Autodesk Inventor part; units mm, degrees
ref_plane "YZ Plane" through (0, 0, 0) normal (1, 0, 0) x (0, 1, 0)
ref_plane "XZ Plane" through (0, 0, 0) normal (0, 1, 0) x (-1, 0, 0)
ref_plane "XY Plane" through (0, 0, 0) normal (0, 0, 1) x (1, 0, 0)
sketch "スケッチ1" plane through (0, 0, 0) normal (0, 0, 1) x (1, 0, 0)
  line L0 (0, 25) -> (-3.75, 25)
  line L1 (-3.75, 25) -> (-3.75, 0)
  line L2 (-3.75, 0) -> (0, 0)
  line L3 (0, 0) -> (0, 25)
  line L4 (0, -5) -> (0, 30)
  line L5 (-4.5, 0) -> (0.75, 0)
  dimension "d2" = 3.75
  dimension "d3" = 25
revolve "回転1" add sketch "スケッチ1" angle 360 about axis through (0, -10, 0) along (0, 1, 0)
sketch "スケッチ3" plane through (0, 25, 0) normal (0, 1, 0) x (1, 0, 0)
  circle A0 centre (0, 0) radius 2.5
  dimension "d5" = 5
extrude "押し出し1" cut sketch "スケッチ3" against normal blind 5
sketch "スケッチ4" plane through (0, 0, 0) normal (0, -1, 0) x (1, 0, 0)
  circle A0 centre (0, 0) radius 3.75
  line L0 (3.75, 3.25) -> (5.75, 3.25)
  line L1 (3.75, -3.25) -> (5.75, -3.25)
  line L2 (5.75, -3.25) -> (5.75, 3.25)
  line L3 (2.7951, 2.5) -> (3.75, 2.5)
  line L4 (-5.65, 0) -> (7.65, 0)
  line L5 (3.75, 3.25) -> (3.75, 2.5)
  line L6 (3.75, 0) -> (3.75, -3.25)
  line L7 (2.7951, -2.5) -> (3.75, -2.5)
  dimension "d9" = 6.5
  dimension "d10" = 2
  dimension "d11" = 2.5
  dimension "d12" = 5
extrude "押し出し2" add sketch "スケッチ4" against normal blind 20 contours L6 L7 A0 | A0 L3 L5 L0 L2 L4 | L4 L2 L1 L6
fillet "フィレット1" radius 0.5 4 edges at (5.75, 10, 3.25) (5.75, 10, -3.25) (3.75, 10, 3.25) (3.75, 10, -3.25)
properties part number "flat_cover_5mm"
Geometry: final body of the model. Coordinates: model frame, mm. A direction names the side the tool comes from. Give positions to 0.01 mm unless a question says otherwise; leave off trailing zeros. Loops run counter-clockwise (first coordinate to the right, second up) from the corner with the lowest first, then second, coordinate; pieces in that order, holes last. Notation, with made-up numbers: (7, 7.5) -> (19, 7.5) arc R18 ccw to (19, 32.5) -> close; hole circle Ø5 at (-15.75, -18). An arc over 180 degrees is marked (long way). Put each result on its own line as item: value.
1. Pin query (flat end, axial travel): P1, Ø0.8, axis at x = 4.5, y = 5.5, coming from the +Z side; P2, Ø2.5, axis at x = 0, z = 1, coming from the +Y side; P3, Ø1.1, axis at x = 4.5, y = 7.5, coming from the -Z side. Return the tip coordinate at first contact, or that it passes through.
Taken from the geometry:
P1: stops at z = 3.25
P2: stops at y = 20
P3: stops at z = -3.25
2. Cut plane D-D (z = 0). Return the cut outline in (x, y).
Taken from the geometry:
outline: (-3.75, 0) -> (5.75, 0) -> (5.75, 20) -> (3.75, 20) -> (3.75, 25) -> (2.5, 25) -> (2.5, 20) -> (-2.5, 20) -> (-2.5, 25) -> (-3.75, 25) -> close
3. Cut plane B-B (x = 0). Return the cut outline in (y, z), plus the area to 4 significant figures.
Taken from the geometry:
outline: (0, -3.75) -> (25, -3.75) -> (25, -2.5) -> (20, -2.5) -> (20, 2.5) -> (25, 2.5) -> (25, 3.75) -> (0, 3.75) -> close
area: 162.5 mm2
4. Cut plane A-A (z = 3). Return the cut outline in (x, y), plus the area to 3 significant figures.
Taken from the geometry:
outline: (-2.25, 0) -> (2.25, 0) -> (2.25, 25) -> (-2.25, 25) -> close; (3.82, 0) -> (5.68, 0) -> (5.68, 20) -> (3.82, 20) -> close
area: 150 mm2
5. Ray query, line 1 along Z through (x, y) = (0, 24); line 2 along Y through (x, z) = (4.75, 2.75). Return the intervals inside material, ascending. Write a range as [from, to].
Taken from the geometry:
line 1: z = [-3.75, -2.5], [2.5, 3.75]
line 2: y = [0, 20]
6. Set-up query: faces 1 (the cylindrical face through (-0.54, 22.54, 2.44)), 2 (the flat face through (3, 10, -2.5)), 3 (the flat face through (3, 10, 2.5)), 4 (the flat face through (5, 10, -3.25)). Return all of +Z, -Z, +X, -X, +Y, -Y with unobstructed straight access to the full face (end or side cutting, diameter ignored); none if empty.
Taken from the geometry:
face 1: +Y
face 2: -Z, +Y, -Y
face 3: +Z, +Y, -Y
face 4: -Z, +X, +Y, -Y
7. Cut plane C-C (y = 17.75). Return the cut outline in (x, z), plus the area to 3 significant figures.
Taken from the geometry:
outline: (2.8, -2.5) -> (3.75, -2.5) -> (3.75, -2.75) arc R0.5 ccw to (4.25, -3.25) -> (5.25, -3.25) arc R0.5 ccw to (5.75, -2.75) -> (5.75, 2.75) arc R0.5 ccw to (5.25, 3.25) -> (4.25, 3.25) arc R0.5 ccw to (3.75, 2.75) -> (3.75, 2.5) -> (2.8, 2.5) arc R3.75 ccw (long way) to start
area: 58.5 mm2
